Source: CAD feature listing. Evaluate the final solid. Frame: model axes, mm. Give positions to 0.01 mm unless a question says otherwise; leave off trailing zeros. Order: outer loops, then holes, each group sorted by start corner. A loop starts at its lowest first (then second) coordinate and runs counter-clockwise, first axis right, second up. Notation, with made-up numbers: (33.25, -28) - (82.25, -28) arc R34 ccw to (82.25, 7) - close; hole circle Ø2 at (-38.75, 57). An arc over 180 degrees is marked (long way). Use CSV: the item, a comma, the result in double quotes.
```python
from build123d import *

# Parameters (mm, degrees)
F1_DEPTH = 25


with BuildPart() as f1:
    # F0 (on Front) → F1 (new body)
    with BuildSketch(Plane.XZ):
        with BuildLine():
            ThreePointArc((-92.43948, 33.851352), (-97.070489, 32.584286), (-99.091926, 28.229347))
            Line((-99.091926, 28.229347), (-99.091926, -26.770653))
            ThreePointArc((-99.091926, -26.770653), (-96.464596, -29.92403), (-92.627565, -31.381369))
            Line((-92.627565, -31.381369), (-42.627565, -31.381369))
            ThreePointArc((-42.627565, -31.381369), (-30.392022, -27.201973), (-18.15648, -31.381369))
            Line((-18.15648, -31.381369), (11.84352, -31.381369))
            ThreePointArc((11.84352, -31.381369), (25.189403, -26.277255), (38.535287, -31.381369))
            Line((38.535287, -31.381369), (68.535287, -31.381369))
            ThreePointArc((68.535287, -31.381369), (73.814491, -30.020555), (77.778015, -26.277255))
            Line((77.778015, -26.277255), (127.778015, -26.277255))
            ThreePointArc((127.778015, -26.277255), (133.003671, -24.585093), (136.245534, -20.150995))
            Line((136.245534, -20.150995), (137.015536, 22.199387))
            ThreePointArc((137.015536, 22.199387), (133.653161, 26.394115), (128.514688, 27.974436))
            Line((128.514688, 27.974436), (78.514688, 27.974436))
            ThreePointArc((78.514688, 27.974436), (74.196713, 32.277135), (68.307743, 33.851352))
            Line((68.307743, 33.851352), (38.307743, 33.851352))
            ThreePointArc((38.307743, 33.851352), (25.901161, 29.538185), (13.49458, 33.851352))
            Line((13.49458, 33.851352), (-16.50542, 33.851352))
            ThreePointArc((-16.50542, 33.851352), (-29.47245, 29.078174), (-42.43948, 33.851352))
            Line((-42.43948, 33.851352), (-92.43948, 33.851352))
        make_face()
    extrude(amount=F1_DEPTH)


solid = f1.part
```
Item 1: Mould query, pull axis X, two halves, no side actions, for faces 1 (the cylindrical face through (133.72, -12.32, 26.35)), 2 (the flat face through (-1, -12, 33.851)), 3 (the flat face through (-99.092, -12, 1)), 4 (the cylindrical face through (26.09, -12.32, 29.54)). Classes: released by +X, released by -X, zero draft, split by the parting line, or undercut.
Filled in:
face 1,"released by +X"
face 2,"zero draft"
face 3,"released by -X"
face 4,"undercut"
Item 2: Section A-A on y = -22.5. Return the cut outline in (x, z), then the cut area to 3 significant figures.
Filled in:
outline,"(-99.09, -26.77) arc R8.09 ccw to (-92.63, -31.38) - (-42.63, -31.38) arc R20 cw to (-18.16, -31.38) - (11.84, -31.38) arc R20 cw to (38.54, -31.38) - (68.54, -31.38) arc R10.92 ccw to (77.78, -26.28) - (127.78, -26.28) arc R8.91 ccw to (136.25, -20.15) - (137.02, 22.2) arc R9.14 ccw to (128.51, 27.97) - (78.51, 27.97) arc R11.8 ccw to (68.31, 33.85) - (38.31, 33.85) arc R20 cw to (13.49, 33.85) - (-16.51, 33.85) arc R20 cw to (-42.44, 33.85) - (-92.44, 33.85) arc R5.7 ccw to (-99.09, 28.23) - close"
area,"14,300 mm2"
Item 3: First-contact query: pin 1 (1.5 mm diameter, centred on y = -16, z = 18.5, fed in from +X); pin 2 (12.5 mm diameter, centred on x = 105.5, y = -13, fed in from -Z); pin 3 (10 mm diameter, centred on y = -10.5, z = -7.5, fed in from +X). Flat tips, straight axial feed; report the tip coordinate or a pass-through.
Filled in:
pin 1,"stops at x = 136.96"
pin 2,"stops at z = -26.28"
pin 3,"stops at x = 136.57"
Item 4: Section B-B on x = 86. Return the cut outline in (y, z).
Filled in:
outline,"(-25, -26.28) - (0, -26.28) - (0, 27.97) - (-25, 27.97) - close"
Item 5: Material intervals for line 1 (Z direction, x = -69, y = -14.25); line 2 (Z direction, x = 120.5, y = -15.25); line 3 (X direction, y = -12.75, z = -1.5), sorted ascending. Write a range as from..to.
Filled in:
line 1,"z = -31.38..33.85"
line 2,"z = -26.28..27.97"
line 3,"x = -99.09..136.58"
Item 6: Section C-C on x = 20. Return the cut outline in (y, z).
Filled in:
outline,"(-25, -26.96) - (0, -26.96) - (0, 30.43) - (-25, 30.43) - close"
